```python
from build123d import *

# Parameters (mm, degrees)
F0_W     = 508
F0_H     = 76.2
F0_R     = 30.2641
F1_DEPTH = 12.7


with BuildPart() as f1:
    # F0 (on Front) → F1 (new body, symmetric)
    with BuildSketch(Plane.XZ):
        with Locations((410.966302, 0)):
            Rectangle(F0_W, F0_H)
        with Locations((220.466302, 0)):
            Circle(F0_R, mode=Mode.SUBTRACT)
        with Locations((601.466302, 0)):
            Circle(F0_R, mode=Mode.SUBTRACT)
    extrude(amount=F1_DEPTH, both=True)


solid = f1.part
```
Model file for the job. Use its own axes, mm. Coordinates: 2 decimals unless noted, no trailing zeros. Write each loop counter-clockwise with the first axis right and the second up, starting at its lowest first coordinate (ties: lowest second). Pieces come first, ordered by that corner, then holes. Notation, with made-up numbers: (60, 30) - (100, 30) arc R24 cw to (100, 60) - close; hole circle Ø9 at (-1, 56.5). An arc over 180 degrees is marked (long way). One line per item, written item: value. Start each with the question number.
1. Mould opens along X. For faces 1 (the flat face through (156.966, 0, -1)), 2 (the flat face through (407, 12.7, 1)), 3 (the cylindrical face through (249.333, 0.178, 9.091)), 4 (the cylindrical face through (629.423, 0.178, -11.591)) say: released by +X, released by -X, zero draft, split by the parting line, or undercut.
2. Slice it at C-C (x = 588.5). Write the cut outline in (y, z), plus the area to 3 significant figures.
3. Probe line 1 (X direction, y = -3.5, z = -12.5); line 2 (X direction, y = 7, z = 17); line 3 (Z direction, x = 215, y = -9.25). List the from-to ranges inside material, lowest first. Write a range as from..to.
4. Slice it at A-A (z = 0). Write the cut outline in (x, y), plus the area to 3 significant figures.
5. Slice it at B-B (y = 4). Write the cut outline in (x, z).
Answers below:
1. face 1: released by -X
1. face 2: zero draft
1. face 3: undercut
1. face 4: undercut
2. outline: (-12.7, -38.1) - (12.7, -38.1) - (12.7, -27.35) - (-12.7, -27.35) - close; (-12.7, 27.35) - (12.7, 27.35) - (12.7, 38.1) - (-12.7, 38.1) - close
2. area: 546 mm^2
3. line 1: x = 156.97..192.9, 248.03..573.9, 629.03..664.97
3. line 2: x = 156.97..195.43, 245.5..576.43, 626.5..664.97
3. line 3: z = -38.1..-29.77, 29.77..38.1
4. outline: (156.97, -12.7) - (190.2, -12.7) - (190.2, 12.7) - (156.97, 12.7) - close; (250.73, -12.7) - (571.2, -12.7) - (571.2, 12.7) - (250.73, 12.7) - close; (631.73, -12.7) - (664.97, -12.7) - (664.97, 12.7) - (631.73, 12.7) - close
4. area: 9,830 mm^2
5. outline: (156.97, -38.1) - (664.97, -38.1) - (664.97, 38.1) - (156.97, 38.1) - close; hole circle Ø60.53 at (220.47, 0); hole circle Ø60.53 at (601.47, 0)
